Geometry check sheet. Reference: the model listing, model coordinates, mm. A direction names the side the tool comes from. Round coordinates to 2 decimals unless told otherwise and drop trailing zeros. Order: outer loops, then holes, each group sorted by start corner. A loop starts at its lowest first (then second) coordinate and runs counter-clockwise, first axis right, second up. Notation, with made-up numbers: M -13,62.5 L 11,62.5 A34 cw 11,101.5 Z; hole C 55,-0.5 d8. An arc over 180 degrees is marked long. Answer as a JSON object with one key per item and string values. Group by question number.
```python
from build123d import *

# Parameters (mm, degrees)
F0_W      = 17
F0_H      = 11
F1_DEPTH  = 11
F3_DEPTH  = 10
F4_W      = 13
F4_H      = 2
F5_DEPTH  = 3
F6_W      = 1.5
F6_H      = 1.5
F7_DEPTH  = 15.001
F8_W      = 2
F8_H      = 2
F9_DEPTH  = 3
F11_DEPTH = 9.501
F12_DEPTH = 1


# Not quite as in the source:
# - a feature names something its author has since deleted; it is built from what else it names


with BuildPart() as f1:
    # F0 (on Top) → F1 (new body)
    with BuildSketch(Plane.XY):
        with Locations((1.3527604751, 0)):
            Rectangle(F0_W, F0_H)
    extrude(amount=F1_DEPTH)

    # F2 (on face) → F3 (cut)
    with BuildSketch(Plane(origin=(0, 5.5, 0), x_dir=(-1, 0, 0), z_dir=(0, 1, 0))):
        Polygon((-7.8527604751, 2), (-1.3527604751, 2), (5.1472395249, 2), (5.1472395249, 5.5), (5.1472395249, 9), (-1.3527604751, 9), (-7.8527604751, 9), (-7.8527604751, 5.5), align=None)
    extrude(amount=-F3_DEPTH, mode=Mode.SUBTRACT)

    # F4 (on face) → F5 (join)
    with BuildSketch(Plane(origin=(0, 5.5, 0), x_dir=(-1, 0, 0), z_dir=(0, 1, 0))):
        with Locations((-1.3527604751, 1)):
            Rectangle(F4_W, F4_H)
    extrude(amount=F5_DEPTH)

    # F6 (on face) → F7 (cut, through all)
    with BuildSketch(Plane.YZ.offset(7.8527604751)):
        with Locations((7, 1)):
            Rectangle(F6_W, F6_H)
    extrude(amount=-F7_DEPTH, mode=Mode.SUBTRACT)

    # F8 (on face) → F9 (join)
    with BuildSketch(Plane.XY.offset(11)):
        with Locations((1.3527604751, 2.5)):
            Rectangle(F8_W, F8_H)
    extrude(amount=F9_DEPTH)

    # F10 (on face) → F11 (cut, through all)
    with BuildSketch(Plane.YZ.offset(2.3527604751)):
        Polygon((2.5089287665, 12.594983913), (1.5, 14), (1.5, 11), align=None)
    extrude(amount=-F11_DEPTH, mode=Mode.SUBTRACT)

    # F12 (add): a face of the model
    f12_faces = [f1.faces().sort_by_distance(p)[0] for p in [
        (1.3527604751, 3.5, 12.5),
    ]]
    extrude(f12_faces, amount=F12_DEPTH)


solid = f1.part
```
1) Release check for a two-part mould opening along Y. For faces 4 (the flat face through (1, -5.5, 5)), 5 (the flat face through (1, 7.75, 1)), 6 (the flat face through (1, 2, 2)) record: +Y half, -Y half, draft (parallel to the pull), parting line (faces both ways), or undercut.
2) Set-up check for faces 1 (the flat face through (1, -4.5, 6)), 2 (the flat face through (2.353, 3, 12)), 3 (the flat face through (1, 7, 1.75)): record each of +Z, -Z, +X, -X, +Y, -Y from which the full face is reachable in a straight line by a thin tool's end or side.
3) Go/stop test with flat-tipped pins: P1, Ø4, axis at x = 5, z = 9, coming from the +Y side; P2, Ø1.6, axis at x = -1, y = 7.5, coming from the +Z side; P3, Ø0.6, axis at y = 6.5, z = 0.5, coming from the -X side. Record where each tip stops, or that it passes through.
4) Sectioned sample at A-A (z = 1). Record the boundary of the cut face in (x, y), then the cut area to 4 significant figures.
5) Thickness scan on line 1 along Z through (x, y) = (4.25, 4); line 2 along X through (y, z) = (2.75, 7); line 3 along Y through (x, z) = (-4.5, 0.5). Record the ranges inside material, lowest first. Write a range as [from, to].
6) Sectioned sample at C-C (x = 1.75). Record the boundary of the cut face in (y, z), then the cut area to 3 significant figures.
7) Sectioned sample at D-D (z = 8.75). Record the boundary of the cut face in (x, y), then the cut area to 3 significant figures.
8) Sectioned sample at B-B (y = 3). Record the boundary of the cut face in (x, z), then the cut area to 3 significant figures.
Final values:
{
 "1": {"face 4": "-Y half", "face 5": "undercut", "face 6": "draft"},
 "2": {"face 1": "+Y", "face 2": "+Z, +X, +Y, -Y", "face 3": "+X, -X"},
 "3": {"P1": "stops at y = 5.5", "P2": "stops at z = 2", "P3": "stops at x = -5.15"},
 "4": {"outline": "M -7.15,-5.5 L 9.85,-5.5 L 9.85,5.5 L 7.85,5.5 L 7.85,6.25 L -5.15,6.25 L -5.15,5.5 L -7.15,5.5 Z; M -5.15,7.75 L 7.85,7.75 L 7.85,8.5 L -5.15,8.5 Z", "area": "206.5 mm^2"},
 "5": {"line 1": "z = [0, 2], [9, 11]", "line 2": "x = [-7.15, -5.15], [7.85, 9.85]", "line 3": "y = [-5.5, 6.25], [7.75, 8.5]"},
 "6": {"outline": "M -5.5,0 L 8.5,0 L 8.5,2 L -4.5,2 L -4.5,9 L 5.5,9 L 5.5,11 L 4.5,11 L 4.5,14 L 1.5,14 L 2.51,12.59 L 1.5,11 L -5.5,11 Z; hole M 6.25,0.25 L 7.75,0.25 L 7.75,1.75 L 6.25,1.75 Z", "area": "62.2 mm^2"},
 "7": {"outline": "M -7.15,-5.5 L 9.85,-5.5 L 9.85,5.5 L 7.85,5.5 L 7.85,-4.5 L -5.15,-4.5 L -5.15,5.5 L -7.15,5.5 Z", "area": "57.0 mm^2"},
 "8": {"outline": "M -7.15,0 L 9.85,0 L 9.85,11 L 2.35,11 L 2.35,14 L 0.35,14 L 0.35,11 L -7.15,11 Z; hole M -5.15,2 L 7.85,2 L 7.85,9 L -5.15,9 Z", "area": "102 mm^2"}
}
